Design review of the part built by this model. Coordinates are the model's own, in mm. Face numbers are marked on the shaded views. A direction names the side the tool comes from. Give positions to 0.01 mm unless a question says otherwise; leave off trailing zeros. Loops run counter-clockwise (first coordinate to the right, second up) from the corner with the lowest first, then second, coordinate; pieces in that order, holes last.
from build123d import *

# Parameters (mm, degrees)
F0_W      = 76.2
F0_H      = 139.7
F1_DEPTH  = 4.7625
F2_W      = 3.175
F2_H      = 139.7
F3_DEPTH  = 28.575
F4_W      = 76.2
F4_H      = 139.7
F5_DEPTH  = 2.921
F6_R      = 11.684
F6_R_2    = 11.049
F7_DEPTH  = 76.2
F6_R_3    = 14.732
F8_DEPTH  = 25.4
F9_R      = 11.43
F10_DEPTH = 25.4
F11_W     = 76.2
F11_H     = 139.7
F12_DEPTH = 4.7625
F13_R     = 14.732
F14_DEPTH = 25.4
F15_W     = 3.175
F15_H     = 38.1
F16_DEPTH = 49.04312
F17_R     = 3.429
F18_DEPTH = 25.4


with BuildPart() as f1:
    # F0 (on Top) → F1 (new body)
    with BuildSketch(Plane.XY):
        Rectangle(F0_W, F0_H)
    extrude(amount=F1_DEPTH)

    # F2 (on face) → F3 (join)
    with BuildSketch(Plane.XY.offset(4.7625)):
        with Locations((-36.5125, 0)):
            Rectangle(F2_W, F2_H)
        with Locations((36.5125, 0)):
            Rectangle(F2_W, F2_H)
    extrude(amount=F3_DEPTH)

    # F4 (on face) → F5 (join)
    with BuildSketch(Plane.XY.offset(33.3375)):
        Rectangle(F4_W, F4_H)
    extrude(amount=F5_DEPTH)

    # F6 (on face) → F7 (cut)
    with BuildSketch(Plane.XY.offset(36.2585)):
        with Locations((0, -8.89)):
            Circle(F6_R)
        with Locations((0, -49.53)):
            Circle(F6_R_2)
    extrude(amount=-F7_DEPTH, mode=Mode.SUBTRACT)

    # F6 (on face) → F8 (cut)
    with BuildSketch(Plane.XY.offset(36.2585)):
        with Locations((0, 31.75)):
            Circle(F6_R_3)
    extrude(amount=-F8_DEPTH, mode=Mode.SUBTRACT)

    # F9 (on face) → F10 (cut)
    with BuildSketch(Plane(origin=(0, 0, 0), x_dir=(1, 0, 0), z_dir=(0, 0, -1))):
        with Locations((0, -34.29)):
            Circle(F9_R)
    extrude(amount=-F10_DEPTH, mode=Mode.SUBTRACT)

    # F11 (on face) → F12 (cut)
    with BuildSketch(Plane(origin=(0, 0, 0), x_dir=(1, 0, 0), z_dir=(0, 0, -1))):
        Rectangle(F11_W, F11_H)
    extrude(amount=-F12_DEPTH, mode=Mode.SUBTRACT)

    # F13 (on face) → F14 (cut)
    with BuildSketch(Plane.XY.offset(36.2585)):
        with Locations((0, -8.89)):
            Circle(F13_R)
    extrude(amount=-F14_DEPTH, mode=Mode.SUBTRACT)

    # F15 (on face) → F16 (cut)
    with BuildSketch(Plane(origin=(0, 0, 4.7625), x_dir=(1, 0, 0), z_dir=(0, 0, -1))):
        with Locations((36.5125, 50.8)):
            Rectangle(F15_W, F15_H)
    extrude(amount=-F16_DEPTH, mode=Mode.SUBTRACT)

    # F17 (on face) → F18 (cut)
    with BuildSketch(Plane.XY.offset(36.2585)):
        with Locations((22.225, -57.15)):
            Circle(F17_R)
    extrude(amount=-F18_DEPTH, mode=Mode.SUBTRACT)


solid = f1.part
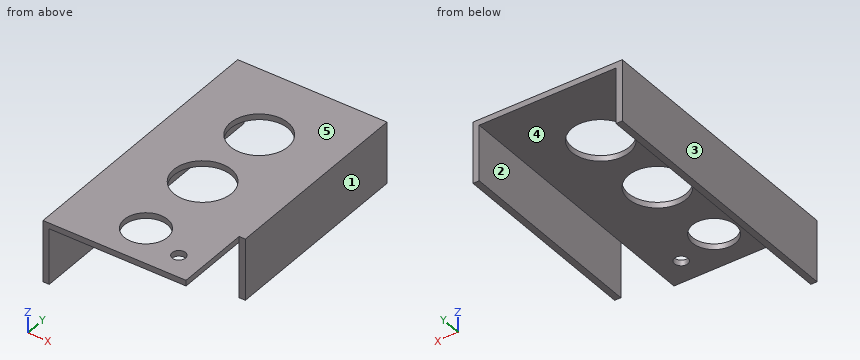
Q1. Tool access review of the marked faces 1 and 2: name each direction out of +Z, -Z, +X, -X, +Y, -Y from which nothing blocks a thin tool from reaching the whole face with its end or side.
Results:
face 1: +Z, -Z, +X, +Y, -Y
face 2: -Z, +Y, -Y
Q2. Take a section at A-A (x = 0). Give the boundary of the cut face in (y, z), plus the area to 3 significant figures.
Results:
outline: (-69.85, 33.34) - (-60.58, 33.34) - (-60.58, 36.26) - (-69.85, 36.26) - close; (-38.48, 33.34) - (-23.62, 33.34) - (-23.62, 36.26) - (-38.48, 36.26) - close; (5.84, 33.34) - (17.02, 33.34) - (17.02, 36.26) - (5.84, 36.26) - close; (46.48, 33.34) - (69.85, 33.34) - (69.85, 36.26) - (46.48, 36.26) - close
area: 171 mm2
Q3. Take a section at C-C (y = -8.89). Give the boundary of the cut face in (x, z) (1 decimal), plus the area to 3 significant figures.
Results:
outline: (-38.1, 4.8) - (-34.9, 4.8) - (-34.9, 33.3) - (-14.7, 33.3) - (-14.7, 36.3) - (-38.1, 36.3) - close; (14.7, 33.3) - (34.9, 33.3) - (34.9, 4.8) - (38.1, 4.8) - (38.1, 36.3) - (14.7, 36.3) - close
area: 318 mm2
Q4. Insertion check: pin 1 (13.5 mm diameter, centred on x = 0, y = -49.53, fed in from -Z); pin 2 (3 mm diameter, centred on x = 20, y = 32, fed in from -Z); pin 3 (8 mm diameter, centred on y = -53.5, z = 26.5, fed in from +X) (3 decimals); pin 4 (2.5 mm diameter, centred on y = -42, z = 35, fed in from +X) (3 decimals). Each pin has a flat end and moves straight along its axis. Give the tip position at first contact, or say it passes through.
Results:
pin 1: passes through
pin 2: stops at z = 33.34
pin 3: stops at x = -34.925
pin 4: stops at x = 34.925
Q5. Wall thickness on line 1 (Y direction, x = 0, z = 35); line 2 (X direction, y = 46, z = 11) (3 decimals); line 3 (Z direction, x = 30, y = 33.5): over which ranges is each line inside the solid? List them lowest first.
Results:
line 1: y = -69.85 to -60.58, -38.48 to -23.62, 5.84 to 17.02, 46.48 to 69.85
line 2: x = -38.1 to -34.925, 34.925 to 38.1
line 3: z = 33.34 to 36.26
Q6. Draft analysis for pull direction X (two halves, no side actions). For the marked faces 3, 4 and 5, state which applies: pulls with the +X half, pulls with the -X half, needs draft (parallel to the pull), parting line crosses it, or undercut.
Results:
face 3: pulls with the -X half
face 4: undercut
face 5: needs draft
Q7. Take a section at D-D (y = -57.15). Give the boundary of the cut face in (x, z) (1 decimal).
Results:
outline: (-38.1, 4.8) - (-34.9, 4.8) - (-34.9, 33.3) - (-8, 33.3) - (-8, 36.3) - (-38.1, 36.3) - close; (8, 33.3) - (18.8, 33.3) - (18.8, 36.3) - (8, 36.3) - close; (25.7, 33.3) - (34.9, 33.3) - (34.9, 36.3) - (25.7, 36.3) - close
Q8. Take a section at B-B (z = 27). Give the boundary of the cut face in (x, y) (3 decimals).
Results:
outline: (-38.1, -69.85) - (-34.925, -69.85) - (-34.925, 69.85) - (-38.1, 69.85) - close; (34.925, -31.75) - (38.1, -31.75) - (38.1, 69.85) - (34.925, 69.85) - close
